```python
from build123d import *

# Parameters (mm, degrees)
F0_R     = 9.525
F1_DEPTH = 25.4
F2_W     = 9.525
F2_H     = 9.525
F3_DEPTH = 25.401
F5_DEPTH = 19.05
F6_R     = 0.508


with BuildPart() as f1:
    # F0 (on Front) → F1 (new body)
    with BuildSketch(Plane.XZ):
        Circle(F0_R)
    extrude(amount=F1_DEPTH)

    # F2 (on face) → F3 (cut, through all)
    with BuildSketch(Plane.XZ.offset(25.4)):
        Rectangle(F2_W, F2_H)
    extrude(amount=-F3_DEPTH, mode=Mode.SUBTRACT)

    # F4 (on face) → F5 (cut)
    with BuildSketch(Plane.XZ.offset(25.4)):
        Polygon((4.577502, -7.940509), (9.165434, -0.006022), (4.587932, 7.934487), (-4.577502, 7.940509), (-9.165434, 0.006022), (-4.587932, -7.934487), align=None)
    extrude(amount=-F5_DEPTH, mode=Mode.SUBTRACT)

    # F6
    f6_edges = [f1.edges().sort_by_distance(p)[0] for p in [
        (-9.525, 0, 0),
    ]]
    fillet(f6_edges, radius=F6_R)


solid = f1.part
```
Model file for the job. Use its own axes, mm. A direction names the side the tool comes from. Coordinates: 2 decimals unless noted, no trailing zeros. Write item = value, one per line. Start each with the question number.
Item 1: Wall check: probe 1 along Y at (x, z) = (-4.5, 6.75); probe 2 along Z at (x, y) = (-8.25, -1.5); probe 3 along Z at (x, y) = (-4, -12.5). Give the ranges that are in metal, low to high. Write a range as [from, to].
Item 2: Drop flat-ended pins along their axis: pin 1 Ø5 at (x, y) = (5.5, -4) entering from +Z; pin 2 Ø5 at (x, z) = (-2.5, 2) entering from -Y; pin 3 Ø2 at (y, z) = (-13, -4) entering from +X. Give the stop position or say it passes through.
Item 3: Pull direction X, two halves, no side cores. Call faces 1 (the face through (-7.559, -12.78, -5.796)), 2 (the face through (6.84, -16.01, -4.03)), 3 (the face through (6, 0, 0)): +X half, -X half, draft (parallel to the pull), parting line (faces both ways), or undercut.
Item 4: 3-axis set-ups, long thin cutter, end or side, ignore diameter. For faces 4 (the face through (-4.762, -3, 0)), 5 (the face through (7, -25.4, -4.2)), 6 (the face through (-6.84, -16.01, 4.03)): which of +Z, -Z, +X, -X, +Y, -Y reach the whole face in a straight line?
Answers:
q1.probe_1 = [-6.35, 0]
q1.probe_2 = [-4.76, 4.76]
q1.probe_3 = [-8.64, -7.93], [7.94, 8.64]
q2.pin_1 = 9.04
q2.pin_2 = -6.35
q2.pin_3 = 9.04
q3.face_1 = parting line
q3.face_2 = undercut
q3.face_3 = draft
q4.face_4 = +Y, -Y
q4.face_5 = +Z, -Z, +X, -X, -Y
q4.face_6 = -Y
